```python
from build123d import *

# Parameters (mm, degrees)
F0_R     = 6.35
F1_DEPTH = 12.7
F2_DEPTH = 3.81
F4_DEPTH = 50.8


with BuildPart() as f1:
    # F0 (on Right) → F1 (new body)
    with BuildSketch(Plane.YZ):
        Polygon((-37.380086, 54.002845), (-70.400086, 20.982845), (-19.600086, 20.982845), (-19.600086, 54.002845), align=None)
        with Locations((-28.490086, 29.872845)):
            Circle(F0_R, mode=Mode.SUBTRACT)
        with Locations((-28.490086, 29.872845)):
            Circle(F0_R)
    extrude(amount=-F1_DEPTH)

    # F0 (on Right) → F2 (cut)
    with BuildSketch(Plane.YZ):
        with Locations((-28.490086, 29.872845)):
            Circle(F0_R)
    extrude(amount=-F2_DEPTH, mode=Mode.SUBTRACT)

    # F3 (on face) → F4 (cut)
    with BuildSketch(Plane(origin=(0, 0, 20.982845), x_dir=(1, 0, 0), z_dir=(0, 0, -1))):
        with BuildLine():
            ThreePointArc((-12.7, 19.600086), (-11.102629, 45.19729), (-6.35, 70.400086))
            Line((-6.35, 70.400086), (-12.7, 70.400086))
            Line((-12.7, 70.400086), (-12.7, 19.600086))
        make_face()
    extrude(amount=-F4_DEPTH, mode=Mode.SUBTRACT)


solid = f1.part
```
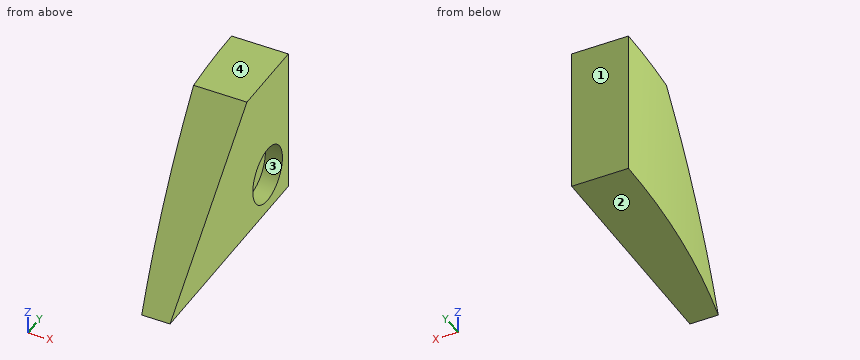
CAD build for the part. Positions are in the model's coordinates, mm. Face numbers are marked on the shaded views. Round coordinates to 2 decimals unless told otherwise and drop trailing zeros. Order: outer loops, then holes, each group sorted by start corner. A loop starts at its lowest first (then second) coordinate and runs counter-clockwise, first axis right, second up. Notation, with made-up numbers: (78, 62.25) - (101, 62.25) arc R14 cw to (101, 85.25) - close; hole circle Ø6 at (19, -32). An arc over 180 degrees is marked (long way). Use CSV: the item, a comma, the result in double quotes. Start each with the question number.
1) Pin check, flat tips, straight feed: pin 1 Ø2 at (x, z) = (-7, 46.5) entering from -Y; pin 2 Ø11.5 at (y, z) = (-28.49, 29.87) entering from +X; pin 3 Ø1.5 at (x, y) = (-9.5, -58.5) entering from +Z. Stop position of each tip, or through.
2) Saw through at D-D (x = -2.25). List the corners of the cut face in (y, z).
3) Saw through at C-C (x = -9.5). List the corners of the cut face in (y, z), and give its area (3 significant figures).
4) Saw through at A-A (y = -33). List the corners of the cut face in (x, z), and give its area (3 significant figures).
5) Wall check: L1, parallel to Y at x = -1.75, z = 32; L2, parallel to Y at x = -5.5, z = 39; L3, parallel to Z at x = -0.75, y = -47. Give the ranges that are in metal, low to high. Write a range as [from, to].
6) Two-plate mould, pull along Z, no slides. Class the marked faces 1, 2, 3 and 4: pulls with the +Z half, pulls with the -Z half, needs draft (parallel to the pull), parting line crosses it, or undercut.
7) Saw through at B-B (z = 25.5). List the corners of the cut face in (x, y).
Values follow:
1,pin 1,"stops at y = -45.88"
1,pin 2,"stops at x = -3.81"
1,pin 3,"stops at z = 33.53"
2,outline,"(-70.4, 20.98) - (-19.6, 20.98) - (-19.6, 54) - (-37.38, 54) - close; hole circle Ø12.7 at (-28.49, 29.87)"
3,outline,"(-55.78, 20.98) - (-19.6, 20.98) - (-19.6, 54) - (-37.38, 54) - (-55.78, 35.6) - close"
3,area,"1,030 mm2"
4,outline,"(-12.26, 20.98) - (0, 20.98) - (0, 25.4) - (-3.81, 25.4) - (-3.81, 34.34) - (0, 34.34) - (0, 54) - (-12.26, 54) - close"
4,area,"371 mm2"
5,L1,"y = [-59.38, -34.47], [-22.51, -19.6]"
5,L2,"y = [-52.38, -19.6]"
5,L3,"z = [20.98, 44.38]"
6,face 1,"needs draft"
6,face 2,"pulls with the -Z half"
6,face 3,"undercut"
6,face 4,"pulls with the +Z half"
7,outline,"(-12.7, -19.6) arc R206.86 ccw to (-7.44, -65.88) - (0, -65.88) - (0, -33.09) - (-3.81, -33.09) - (-3.81, -23.89) - (0, -23.89) - (0, -19.6) - close"
